Verification items for this drawing (mm, ordinates from the low corner). A direction names the side the tool comes from. Round coordinates to 2 decimals unless told otherwise and drop trailing zeros. Loops run counter-clockwise (first coordinate to the right, second up) from the corner with the lowest first, then second, coordinate; pieces in that order, holes last. Notation, with made-up numbers: M -19.75,89.5 L 27.25,89.5 A31 ccw 27.25,122.5 Z; hole C 59,47 d9. An arc over 180 degrees is marked long. Write item = value, one per line. Start each with the question number.
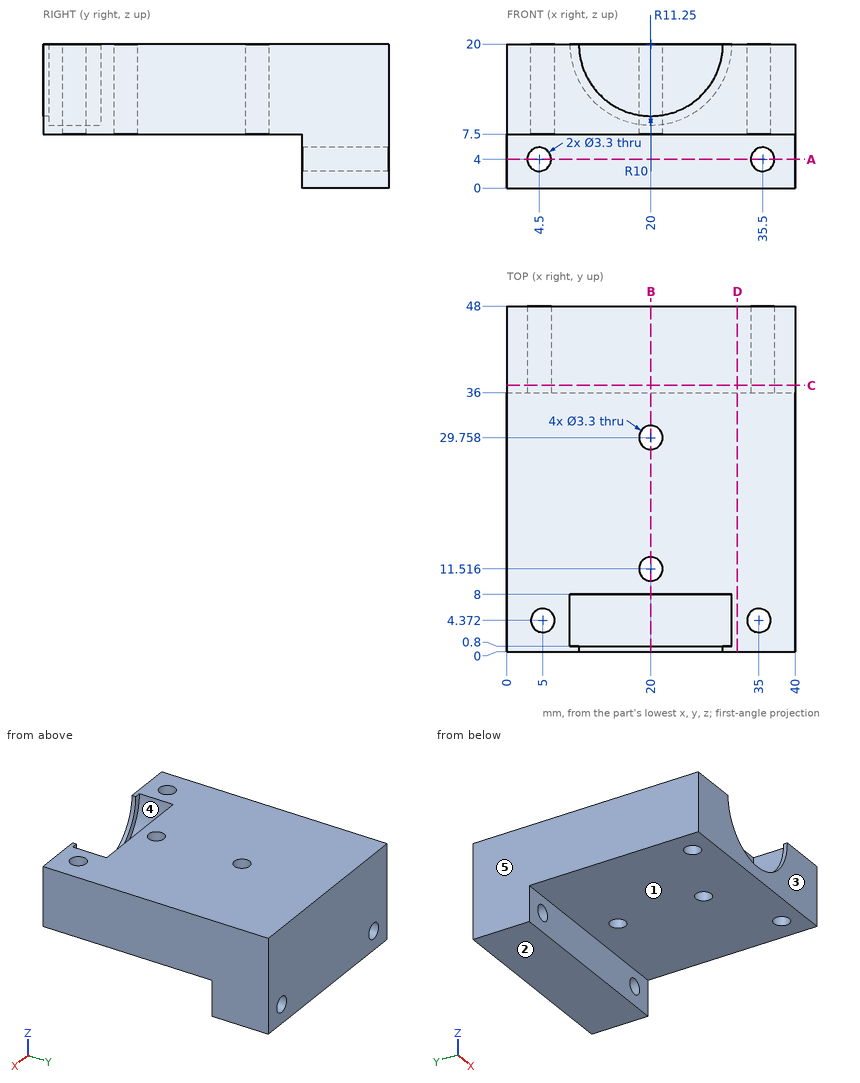
1. Tool access check on the marked faces 1 and 2. Record the directions out of +Z, -Z, +X, -X, +Y, -Y that give a thin tool (end or side, any length) a straight path to the whole face; none if there is none.
2. Mould release check, pull along Y, two halves, no side actions. Record for the marked faces 3, 4 and 5: pulls with the +Y half, pulls with the -Y half, needs draft (parallel to the pull), parting line crosses it, or undercut.
3. Section check A-A, the plane z = 4. Enter the section's corners in (x, y).
4. Section check C-C, the plane y = 37. Enter the section's corners in (x, z), and give its area (3 significant figures).
5. Section check D-D, the plane x = 32. Enter the section's corners in (y, z).
6. Gauge pin test, flat ends, axial feed: P1, Ø2, axis at x = 35, y = 4.37, coming from the +Z side; P2, Ø6, axis at x = 12.5, y = 5, coming from the -Z side; P3, Ø4, axis at x = 17, z = 4, coming from the -Y side; P4, Ø3.5, axis at x = 18.5, z = 13, coming from the -Y side. Record the tip position at first contact, or that the pin passes through.
7. Section check B-B, the plane x = 20. Give the number of separate pieces and of enclosed holes in the cut face.
8. Thickness scan on line 1 (X direction, y = 41, z = 4); line 2 (Y direction, x = 5, z = 17.75); line 3 (X direction, y = 3, z = 15.25) (1 decimal). Record the ranges inside material, lowest first.
Computed values:
q1.face_1 = -Z, +X, -X, -Y
q1.face_2 = -Z, +X, -X, +Y, -Y
q2.face_3 = pulls with the -Y half
q2.face_4 = undercut
q2.face_5 = needs draft
q3.outline = M 0,36 L 2.85,36 L 2.85,48 L 0,48 Z; M 6.15,36 L 33.85,36 L 33.85,48 L 6.15,48 Z; M 37.15,36 L 40,36 L 40,48 L 37.15,48 Z
q4.outline = M 0,0 L 40,0 L 40,20 L 0,20 Z; hole C 4.5,4 d3.3; hole C 35.5,4 d3.3
q4.area = 783 mm2
q5.outline = M 0,7.5 L 36,7.5 L 36,0 L 48,0 L 48,20 L 0,20 Z
q6.P1 = through
q6.P2 = 7.5
q6.P3 = 36
q6.P4 = 8
q7.separate_pieces = 3
q7.enclosed_holes = 0
q8.line_1 = 0 to 2.85, 6.15 to 33.85, 37.15 to 40
q8.line_2 = 0 to 2.72, 6.02 to 48
q8.line_3 = 0 to 4.1, 5.9 to 9.8, 30.2 to 34.1, 35.9 to 40
